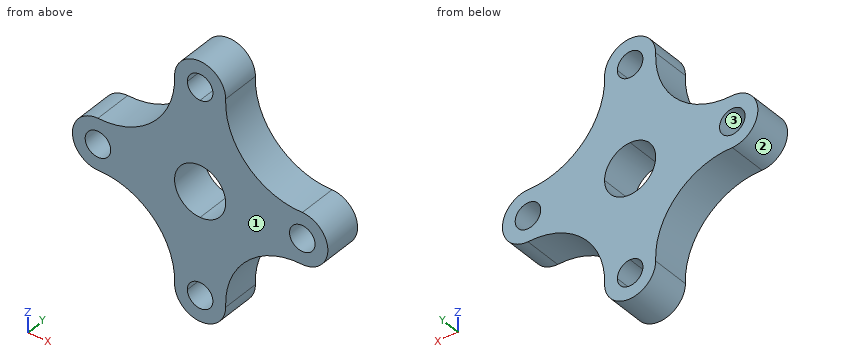
```python
from build123d import *

# Parameters (mm, degrees)
F0_R     = 6.35
F1_DEPTH = 19.05


with BuildPart() as f1:
    # F0 (on Front) → F1 (new body)
    with BuildSketch(Plane.XZ):
        with Locations((-50.8, 0)):
            Circle(F0_R)
        with BuildLine():
            ThreePointArc((44.45, 0), (50.8, -6.35), (57.15, 0))
            ThreePointArc((57.15, 0), (50.8, 6.35), (44.45, 0))
        make_face()
        with BuildLine():
            ThreePointArc((-12.7, 50.8), (-23.358147, 23.358147), (-50.8, 12.7))
            ThreePointArc((-50.8, 12.7), (-63.5, 0), (-50.8, -12.7))
            ThreePointArc((-50.8, -12.7), (-23.358147, -23.358147), (-12.7, -50.8))
            ThreePointArc((-12.7, -50.8), (0, -63.5), (12.7, -50.8))
            ThreePointArc((12.7, -50.8), (23.358147, -23.358147), (50.8, -12.7))
            ThreePointArc((50.8, -12.7), (63.5, 0), (50.8, 12.7))
            ThreePointArc((50.8, 12.7), (23.358147, 23.358147), (12.7, 50.8))
            ThreePointArc((12.7, 50.8), (0, 63.5), (-12.7, 50.8))
        make_face()
        with BuildLine():
            ThreePointArc((-6.35, -50.8), (-4.490128, -46.309872), (0, -44.45))
            ThreePointArc((0, -44.45), (4.490128, -46.309872), (6.35, -50.8))
            ThreePointArc((6.35, -50.8), (0, -57.15), (-6.35, -50.8))
        make_face(mode=Mode.SUBTRACT)
        with Locations((-50.8, 0)):
            Circle(F0_R, mode=Mode.SUBTRACT)
        with BuildLine():
            ThreePointArc((0, 12.7), (8.980256, 8.980256), (12.7, 0))
            ThreePointArc((12.7, 0), (8.980256, -8.980256), (0, -12.7))
            ThreePointArc((0, -12.7), (-12.7, 0), (0, 12.7))
        make_face(mode=Mode.SUBTRACT)
        with BuildLine():
            ThreePointArc((44.45, 0), (50.8, 6.35), (57.15, 0))
            ThreePointArc((57.15, 0), (50.8, -6.35), (44.45, 0))
        make_face(mode=Mode.SUBTRACT)
        with BuildLine():
            ThreePointArc((6.35, 50.8), (4.490128, 46.309872), (0, 44.45))
            ThreePointArc((0, 44.45), (-4.490128, 46.309872), (-6.35, 50.8))
            ThreePointArc((-6.35, 50.8), (0, 57.15), (6.35, 50.8))
        make_face(mode=Mode.SUBTRACT)
    extrude(amount=F1_DEPTH)


solid = f1.part
```
Source: CAD feature listing. Evaluate the final solid. Frame: model axes, mm. Face numbers are marked on the shaded views. Give positions to 0.01 mm unless a question says otherwise; leave off trailing zeros. Loops run counter-clockwise (first coordinate to the right, second up) from the corner with the lowest first, then second, coordinate; pieces in that order, holes last. Notation, with made-up numbers: (-33.5, 37) -> (11.5, 37) arc R24 cw to (11.5, 69) -> close; hole circle Ø5 at (49.25, 38.25). An arc over 180 degrees is marked (long way). Use a Markdown table: item, result. Add a question column.
(1) Pull-direction query (X, two-part tool) for the marked faces 1, 2 and 3; classes: +X half, -X half, draft (parallel to the pull), parting line (faces both ways), or undercut.
(2) Section query B-B (z = -17). Output: boundary loops of the cut face in (x, y), then the cut area to 3 significant figures.
(3) First-contact query: pin 1 Ø5 at (x, y) = (23, -12) entering from -Z; pin 2 Ø16.5 at (x, z) = (50.8, 0) entering from -Y; pin 3 Ø8 at (x, y) = (5.5, -15.5) entering from +Z; pin 4 Ø2 at (y, z) = (-12, 12.5) entering from -X. Flat tips, straight axial feed; report the tip coordinate or a pass-through.
(4) Section query C-C (x = 14.5). Output: boundary loops of the cut face in (y, z).
(5) Ray query, line 1 (Z direction, x = -3, y = -9.5); line 2 (Z direction, x = 50.8, y = -11.75); line 3 (Z direction, x = 2.5, y = -16). Return the intervals inside material, ascending.
(6) Section query A-A (y = -7.75). Count the separate pieces of the cut face and the enclosed holes in it, then the cut area to 3 significant figures.
Checked values:
| question | item | result |
|---|---|---|
| 1 | face 1 | draft |
| 1 | face 2 | -X half |
| 1 | face 3 | undercut |
| 2 | outline | (-31.92, -19.05) -> (31.92, -19.05) -> (31.92, 0) -> (-31.92, 0) -> close |
| 2 | area | 1,220 mm^2 |
| 3 | pin 1 | z = -26.57 |
| 3 | pin 2 | y = -19.05 |
| 3 | pin 3 | z = 63.41 |
| 3 | pin 4 | x = -56.19 |
| 4 | outline | (-19.05, -37.74) -> (0, -37.74) -> (0, 37.74) -> (-19.05, 37.74) -> close |
| 5 | line 1 | -63.14 to -56.4, -45.2 to -12.34, 12.34 to 45.2, 56.4 to 63.14 |
| 5 | line 2 | -12.7 to -6.35, 6.35 to 12.7 |
| 5 | line 3 | -63.25 to -56.64, -44.96 to -12.45, 12.45 to 44.96, 56.64 to 63.25 |
| 6 | separate pieces | 1 |
| 6 | enclosed holes | 5 |
| 6 | area | 5,650 mm^2 |
